Here's how the part is built. I have some questions about the finished solid (model axes, mm). Face numbers are marked on the shaded views. A direction names the side the tool comes from. Coordinates: 2 decimals unless noted, no trailing zeros. Write each loop counter-clockwise with the first axis right and the second up, starting at its lowest first coordinate (ties: lowest second). Pieces come first, ordered by that corner, then holes. Notation, with made-up numbers: M 61.5,61 L 115.5,61 A8 cw 115.5,74 Z; hole C 51,53 d6. An arc over 180 degrees is marked long. Use one line per item in the form item = value. Start each with the question number.
1. I'm going to push flat-ended pins straight in: pin 1 Ø3 at (y, z) = (2.5, -4.5) entering from +X; pin 2 Ø1.9 at (x, y) = (-1.5, 4.5) entering from +Z. Where does each tip first touch, or does it pass through?
2. Thinking about a two-plate mould opening in X: for the marked faces 4, 5 and 6, which applies, released by +X, released by -X, zero draft, split by the parting line, or undercut?
3. I want a section at B-B, the plane z = -0.25. List the corners of the cut face in (x, y) for me.
4. I want a section at C-C, the plane y = 5.75. List the corners of the cut face in (x, z) for me.
5. I want a section at D-D, the plane z = -8.5. List the corners of the cut face in (x, y) for me.
6. Please list where these lines run through material, in increasing order: line 1 along Y through (x, z) = (-8.75, 4); line 2 along X through (y, z) = (1.75, 6.5); line 3 along X through (y, z) = (3, 0). Write a range as [from, to].
7. On a 3-axis mill with a long thin cutter (end or side, diameter ignored), from which of +Z, -Z, +X, -X, +Y, -Y can I reach the whole of each face in a straight line? I mean the marked faces 1, 2 and 3. Say none if no direction works.
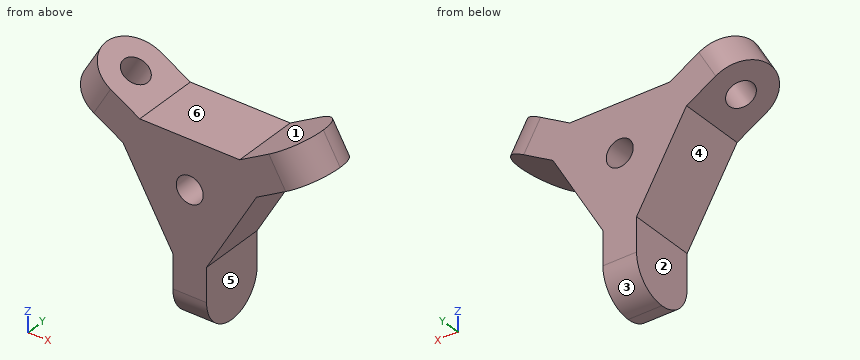
from build123d import *

# Parameters (mm, degrees)
SKETCH1_R           = 1.27
SKETCH1_W           = 3.175
SKETCH1_H           = 6.35
BOSS_EXTRUDE1_DEPTH = 6.35
CUT_EXTRUDE1_REACH  = 21.921
SKETCH2_R           = 1.27
FILLET1_R           = 3.175


with BuildPart() as part:
    # Sketch1 → Boss-Extrude1 (new body)
    # profile 1 of 4: a face of its own
    with BuildSketch(Plane(origin=(0, 0, 0), x_dir=(1, 0, 0), z_dir=(0, 1, 0))):
        Polygon((4.705511314, -4.549815329), (6.293011314, -1.800184671), (1.5875, 6.35), (-1.5875, 6.35), (-6.293011314, -1.800184671), (-4.705511314, -4.549815329), align=None)
        with Locations(Location((0, 0, 0), (0, 0, 270))):
            Circle(SKETCH1_R, mode=Mode.SUBTRACT)
    # profile 2 of 4: a face of its own
    with BuildSketch(Plane(origin=(0, 0, 0), x_dir=(1, 0, 0), z_dir=(0, 1, 0))):
        Polygon((-11.792272628, -4.975184671), (-10.204772628, -7.724815329), (-4.705511314, -4.549815329), (-6.293011314, -1.800184671), align=None)
    # profile 3 of 4: a face of its own
    with BuildSketch(Plane(origin=(0, 0, 0), x_dir=(1, 0, 0), z_dir=(0, 1, 0))):
        Polygon((10.204772628, -7.724815329), (11.792272628, -4.975184671), (6.293011314, -1.800184671), (4.705511314, -4.549815329), align=None)
    # profile 4 of 4: a face of its own
    with BuildSketch(Plane(origin=(0, 0, 0), x_dir=(1, 0, 0), z_dir=(0, 1, 0))):
        with Locations((0, 9.525)):
            Rectangle(SKETCH1_W, SKETCH1_H)
    extrude(amount=BOSS_EXTRUDE1_DEPTH)

    # Sketch2 → Cut-Extrude1 (cut, up to next)
    with BuildSketch(Plane(origin=(0.79375, 0, 1.374815329), x_dir=(0.8660254037844384, 0, -0.5000000000000006), z_dir=(0.5000000000000006, 0, 0.8660254037844384)), mode=Mode.PRIVATE) as cut_extrude1_sk1:
        with Locations((-9.525, 3.175)):
            Circle(SKETCH2_R)
    cut_extrude1_tool1 = extrude(cut_extrude1_sk1.sketch, amount=-CUT_EXTRUDE1_REACH, mode=Mode.PRIVATE) & part.part
    add(cut_extrude1_tool1.solids().sort_by_distance((-7.455142, 3.175, 6.137315))[0], mode=Mode.SUBTRACT)

    # Fillet1
    fillet1_edges = [part.edges().sort_by_distance(p)[0] for p in [
        (0, 0, -12.7),
        (0, 6.35, -12.7),
        (10.998522628, 0, 6.35),
        (10.998522628, 6.35, 6.35),
        (-10.998522628, 0, 6.35),
        (-10.998522628, 6.35, 6.35),
    ]]
    fillet(fillet1_edges, radius=FILLET1_R - 0.0001)  # a hair under: the kernel refuses the full size


solid = part.part
Answer list:
q1.pin_1 = 3.52
q1.pin_2 = 4.55
q2.face_4 = released by -X
q2.face_5 = released by +X
q2.face_6 = undercut
q3.outline = M -5.11,0 L -1.25,0 L -1.25,6.35 L -5.11,6.35 Z; M 1.25,0 L 5.11,0 L 5.11,6.35 L 1.25,6.35 Z
q4.outline = M -10.65,4.32 L -6.29,1.8 L -1.59,-6.35 L -1.59,-11.38 L 1.59,-11.38 L 1.59,-6.35 L 6.29,1.8 L 10.65,4.32 L 9.06,7.07 L 4.71,4.55 L -4.71,4.55 L -9.06,7.07 Z; hole C 0,0 d2.54
q5.outline = M -1.59,0 L 1.59,0 L 1.59,6.35 L -1.59,6.35 Z
q6.line_1 = [0, 1.91], [4.44, 6.35]
q6.line_2 = [-10.52, -8.08], [8.08, 10.52]
q6.line_3 = [-5.25, -1.27], [1.27, 5.25]
q7.face_1 = +Z, +Y, -Y
q7.face_2 = -Z, -X, +Y, -Y
q7.face_3 = -Z, +X, -X, +Y
